Job drawing, mm, ordinate dimensions from the low corner. One solid piece. Round coordinates to 2 decimals unless told otherwise and drop trailing zeros. Write each loop counter-clockwise with the first axis right and the second up, starting at its lowest first coordinate (ties: lowest second). Pieces come first, ordered by that corner, then holes. Notation, with made-up numbers: M 10.25,-4.5 L 64.25,-4.5 A25 cw 64.25,21.5 Z; hole C 28.5,43.5 d11. An arc over 180 degrees is marked long. One line per item, written item: value. Start each with the question number.
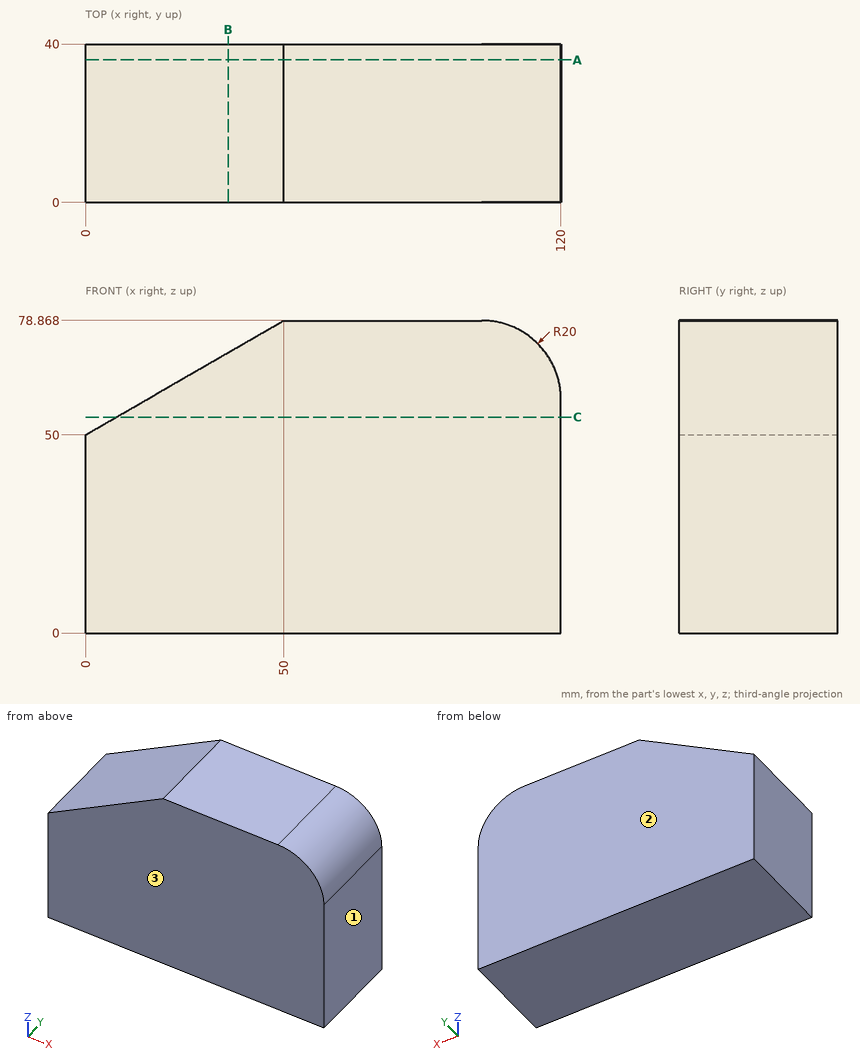
Item 1: Cut at B-B, the plane x = 36. Write the cut outline in (y, z) (1 decimal), plus the area to 3 significant figures.
Item 2: Cut at C-C, the plane z = 54.5. Write the cut outline in (x, y) (1 decimal).
Item 3: Two-plate mould, pull along Y, no slides. Class the marked faces 1, 2 and 3: pulls with the +Y half, pulls with the -Y half, needs draft (parallel to the pull), parting line crosses it, or undercut.
Item 4: Cut at A-A, the plane y = 36. Write the cut outline in (x, z), plus the area to 3 significant figures.
Item 5: Drill centre lines: line 1 (Z direction, x = 6.5, y = 29.5); line 2 (Z direction, x = 38, y = 14.5); line 3 (X direction, y = 25, z = 57.5). Where is each one in solid material? Low to high.
Computed values:
1. outline: M 0,0 L 40,0 L 40,70.8 L 0,70.8 Z
1. area: 2,830 mm2
2. outline: M 7.8,0 L 120,0 L 120,40 L 7.8,40 Z
3. face 1: needs draft
3. face 2: pulls with the +Y half
3. face 3: pulls with the -Y half
4. outline: M 0,0 L 120,0 L 120,58.87 A20 ccw 100,78.87 L 50,78.87 L 0,50 Z
4. area: 8,660 mm2
5. line 1: z = 0 to 53.75
5. line 2: z = 0 to 71.94
5. line 3: x = 12.99 to 120
